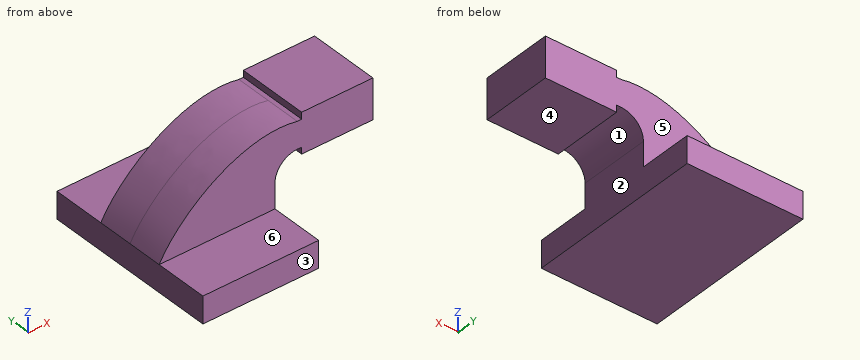
```python
from build123d import *

# Parameters (mm, degrees)
F1_DEPTH = 63.5
F0_W     = 25.4
F0_H     = 19.05
F0_H_2   = 4.7498
F0_H_3   = 4.7752
F2_DEPTH = 25.4


with BuildPart() as f1:
    # F0 (on Front) → F1 (new body, symmetric)
    with BuildSketch(Plane.XZ):
        Polygon((-41.275, 9.525), (-41.275, -9.525), (41.275, -9.525), (41.275, 9.525), (22.225, 9.525), align=None)
    extrude(amount=F1_DEPTH, both=True)

    # F0 (on Front) → F2 (join, symmetric)
    with BuildSketch(Plane.XZ):
        Polygon((-41.275, 9.525), (-41.275, -9.525), (41.275, -9.525), (41.275, 9.525), (22.225, 9.525), align=None)
        with BuildLine():
            add(Edge.make_bspline(
                [(-41.275, 9.525), (-26.6867671162, 36.4819094539), (17.2914229333, 70.0652599335), (57.15, 61.9252)],
                knots=[0, 0, 0, 0, 111.5045361635, 111.5045361635, 111.5045361635, 111.5045361635], degree=3))
            Line((-41.275, 9.525), (22.225, 9.525))
            Line((22.225, 9.525), (22.225, 27.0002))
            ThreePointArc((22.225, 27.0002), (32.4542956671, 51.6959043329), (57.15, 61.9252))
        make_face()
        with BuildLine():
            Line((22.225, 9.525), (41.275, 9.525))
            Line((41.275, 9.525), (41.275, 27.0002))
            ThreePointArc((41.275, 27.0002), (45.9246798487, 38.2255201513), (57.15, 42.8752))
            Line((57.15, 42.8752), (60.325, 42.8752))
            Line((60.325, 42.8752), (60.325, 61.9252))
            Line((60.325, 61.9252), (57.15, 61.9252))
            ThreePointArc((57.15, 61.9252), (32.4542956671, 51.6959043329), (22.225, 27.0002))
            Line((22.225, 27.0002), (22.225, 9.525))
        make_face()
        with Locations((73.025, 52.4002)):
            Rectangle(F0_W, F0_H)
        with Locations((73.025, 64.3001)):
            Rectangle(F0_W, F0_H_2)
        with Locations((73.025, 40.4876)):
            Rectangle(F0_W, F0_H_3)
        Polygon((85.725, 66.675), (85.725, 61.9252), (85.725, 42.8752), (85.725, 38.1), (111.125, 38.1), (111.125, 66.675), align=None)
    extrude(amount=F2_DEPTH, both=True)


solid = f1.part
```
Can you work these out from the model? Positions are in its coordinate system, mm. Face numbers are marked on the shaded views. A direction names the side the tool comes from. Round coordinates to 2 decimals unless told otherwise and drop trailing zeros. Loops run counter-clockwise (first coordinate to the right, second up) from the corner with the lowest first, then second, coordinate; pieces in that order, holes last. Notation, with made-up numbers: (3, 52) -> (32, 52) arc R26 ccw to (32, 76) -> close; hole circle Ø9 at (-21.5, 87). An arc over 180 degrees is marked (long way). One line per item, written item: value. Start each with the question number.
1. For the marked faces 4, 5 and 6, which set-ups out of +Z, -Z, +X, -X, +Y, -Y let a thin tool reach every point of the face, with its end or its side?
2. For pin 1 (3.5 mm diameter, centred on x = 59.5, y = 11, fed in from -Z); pin 2 (18.5 mm diameter, centred on y = 27.5, z = 5, fed in from +X) (3 decimals); pin 3 (1 mm diameter, centred on x = 58, y = -12, fed in from +Z), each with a flat end and sliding along its axis, tell me the tip position at first contact or that it passes through.
3. If I drill on probe 1 along Y at (x, z) = (103.5, 44.5); probe 2 along Z at (x, y) = (1.5, -35) (3 decimals); probe 3 along X at (y, z) = (-54, -5) (3 decimals), over which ranges is the centre line in solid material (lowest first)?
4. If we section it at B-B, the plane y = 30.5: Write out the boundary of the cut face in (x, z) (3 decimals).
5. If we section it at A-A, the plane x = 87: Write out the boundary of the cut face in (y, z) (3 decimals), then the cut area to 3 significant figures.
6. If we mould it in two halves opening along X, with no side actions, what happens to the marked faces 1, 2 and 3? For each: pulls with the +X half, pulls with the -X half, needs draft (parallel to the pull), parting line crosses it, or undercut.
Calculated:
1. face 4: -Z, +X, +Y, -Y
1. face 5: +Z, +X, -X, +Y
1. face 6: +Z, +X, -X, -Y
2. pin 1: stops at z = 38.1
2. pin 2: stops at x = 41.275
2. pin 3: stops at z = 61.93
3. probe 1: y = -25.4 to 25.4
3. probe 2: z = -9.525 to 9.525
3. probe 3: x = -41.275 to 41.275
4. outline: (-41.275, -9.525) -> (41.275, -9.525) -> (41.275, 9.525) -> (-41.275, 9.525) -> close
5. outline: (-25.4, 38.1) -> (25.4, 38.1) -> (25.4, 66.675) -> (-25.4, 66.675) -> close
5. area: 1,450 mm²
6. face 1: undercut
6. face 2: pulls with the +X half
6. face 3: needs draft
